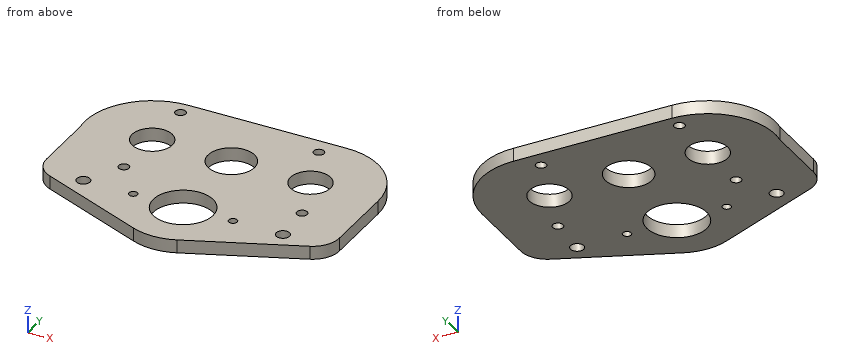
from build123d import *

# Parameters (mm, degrees)
SKETCH1_R           = 14.2875
SKETCH1_R_2         = 9.5885
SKETCH1_R_3         = 11.1125
SKETCH1_R_4         = 3.175
SKETCH1_R_5         = 2.0193
SKETCH1_R_6         = 2.4892
BOSS_EXTRUDE1_DEPTH = 3.175


with BuildPart() as part:
    # Sketch1 → Boss-Extrude1 (new, symmetric)
    with BuildSketch(Plane.XY):
        with BuildLine():
            Line((-37.779325, 75.5142), (37.779325, 75.5142))
            ThreePointArc((37.779325, 75.5142), (60.589175548, 66.066050548), (70.037325, 43.2562))
            Line((70.037325, 43.2562), (70.037325, 8.459528855))
            ThreePointArc((70.037325, 8.459528855), (67.907089191, 1.418926257), (62.231012411, -3.259763936))
            Line((62.231012411, -3.259763936), (10.399085748, -24.903497181))
            ThreePointArc((10.399085748, -24.903497181), (-4.3461e-05, -26.9875), (-10.399165957, -24.903463688))
            Line((-10.399165957, -24.903463688), (-61.816293797, -3.432745712))
            ThreePointArc((-61.816293797, -3.432745712), (-67.49234417, 1.245945741), (-69.622568641, 8.286531317))
            Line((-69.622568641, 8.286531317), (-69.622568641, 38.1))
            ThreePointArc((-69.622568641, 38.1), (-62.344618237, 64.163732906), (-37.779325, 75.5142))
        make_face()
        Circle(SKETCH1_R, mode=Mode.SUBTRACT)
        with Locations((-37.779325, 43.2562)):
            Circle(SKETCH1_R_2, mode=Mode.SUBTRACT)
        with Locations((37.779325, 43.2562)):
            Circle(SKETCH1_R_2, mode=Mode.SUBTRACT)
        with Locations((0, 43.2562)):
            Circle(SKETCH1_R_3, mode=Mode.SUBTRACT)
        with Locations((-47.625, 0)):
            Circle(SKETCH1_R_4, mode=Mode.SUBTRACT)
        with Locations((47.625, 0)):
            Circle(SKETCH1_R_4, mode=Mode.SUBTRACT)
        with Locations((-23.8125, 0)):
            Circle(SKETCH1_R_5, mode=Mode.SUBTRACT)
        with Locations((23.8125, 0)):
            Circle(SKETCH1_R_5, mode=Mode.SUBTRACT)
        with Locations((-37.779325, 68.6562)):
            Circle(SKETCH1_R_6, mode=Mode.SUBTRACT)
        with Locations((-37.779325, 17.8562)):
            Circle(SKETCH1_R_6, mode=Mode.SUBTRACT)
        with Locations((46.46663664, 19.388007432)):
            Circle(SKETCH1_R_6, mode=Mode.SUBTRACT)
        with Locations((29.09201336, 67.124392568)):
            Circle(SKETCH1_R_6, mode=Mode.SUBTRACT)
    extrude(amount=BOSS_EXTRUDE1_DEPTH, both=True)


solid = part.part
For this review, take the finished solid that the model builds, in its own axes (mm). Give positions to 0.01 mm unless a question says otherwise; leave off trailing zeros. Loops run counter-clockwise (first coordinate to the right, second up) from the corner with the lowest first, then second, coordinate; pieces in that order, holes last.
Item 1: For line 1 along Y through (x, z) = (6, 0); line 2 along Y through (x, z) = (0, -0.25); line 3 along X through (y, z) = (46.5, -0.25), list the stretches that pass through material, from the lowest coordinate up.
Item 2: Take a section at B-B, the plane y = 0. Give the number of separate pieces and of enclosed holes in the cut face, and give its area (3 significant figures).
Item 3: Take a section at C-C, the plane x = 42. State the section outline as (y, z) points (3 decimals), and give its area (3 significant figures).
Item 4: Take a section at D-D, the plane y = -11.5. State the section outline as (x, z) points (3 decimals), and give its area (3 significant figures).
Item 5: Take a section at A-A, the plane x = 0. State the section outline as (y, z) points (1 decimal).
Item 6: Insertion check: pin 1 (3 mm diameter, centred on y = 30, z = 1.5, fed in from -X); pin 2 (3 mm diameter, centred on y = 52, z = 2, fed in from -X). Each pin has a flat end and moves straight along its axis. Give the tip position at first contact, or say it passes through.
Calculated:
1. line 1: y = -26.31 to -12.97, 12.97 to 33.9, 52.61 to 75.51
1. line 2: y = -26.99 to -14.29, 14.29 to 32.14, 54.37 to 75.51
1. line 3: x = -69.87 to -46.8, -28.76 to -10.63, 10.63 to 28.76, 46.8 to 69.87
2. separate pieces: 6
2. enclosed holes: 0
2. area: 533 mm2
3. outline: (-11.708, -3.175) - (34.647, -3.175) - (34.647, 3.175) - (-11.708, 3.175) - close; (51.866, -3.175) - (75.237, -3.175) - (75.237, 3.175) - (51.866, 3.175) - close
3. area: 443 mm2
4. outline: (-42.497, -3.175) - (-8.478, -3.175) - (-8.478, 3.175) - (-42.497, 3.175) - close; (8.478, -3.175) - (42.497, -3.175) - (42.497, 3.175) - (8.478, 3.175) - close
4. area: 432 mm2
5. outline: (-27, -3.2) - (-14.3, -3.2) - (-14.3, 3.2) - (-27, 3.2) - close; (14.3, -3.2) - (32.1, -3.2) - (32.1, 3.2) - (14.3, 3.2) - close; (54.4, -3.2) - (75.5, -3.2) - (75.5, 3.2) - (54.4, 3.2) - close
6. pin 1: stops at x = -69.62
6. pin 2: stops at x = -69.21
